Could you check a few things on this drawing? It's one solid part, dimensions in mm from its lowest x, y, z. Round coordinates to 2 decimals unless told otherwise and drop trailing zeros. Write each loop counter-clockwise with the first axis right and the second up, starting at its lowest first coordinate (ties: lowest second). Pieces come first, ordered by that corner, then holes. Notation, with made-up numbers: M -36.5,71 L -4.5,71 A18 cw -4.5,99 Z; hole C 25,30 d11. An arc over 180 degrees is marked long. One line per item, written item: value. Start each with the question number.
(1) I'm going to push a flat-ended pin straight in: pin 1 Ø1 at (x, y) = (15, 1) entering from +Z. Where does the tip first touch, or does it pass through?
(2) I want a section at A-A on x = 26. Please give me the cut outline in (y, z).
(3) If I drill on L1, parallel to Y at x = 20.5, z = 3.6 (3 decimals); L2, parallel to Z at x = 20, y = 2.7, over which ranges is the centre line in solid material (lowest first)?
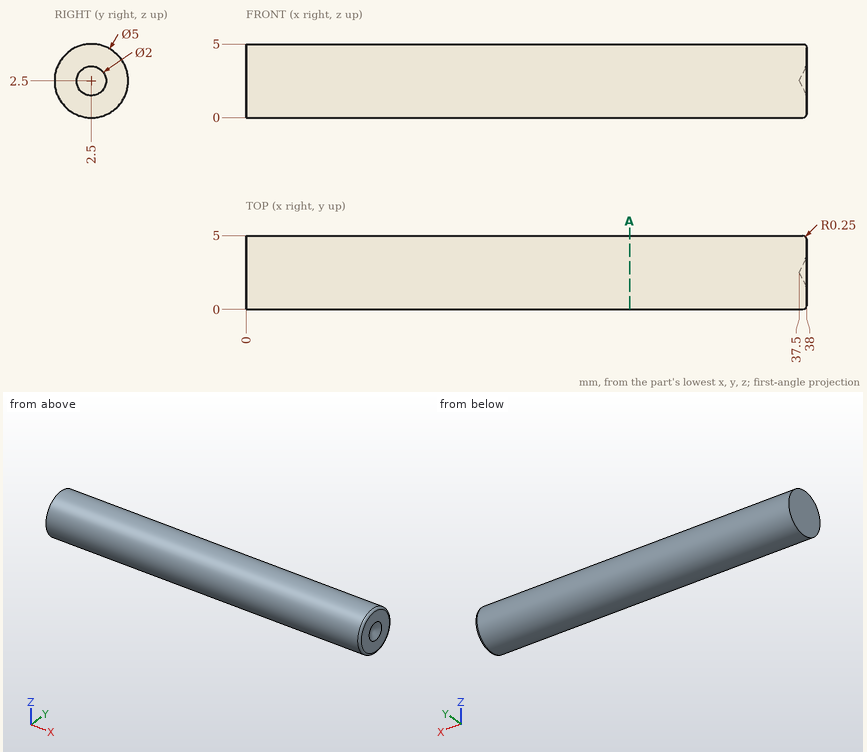
Found:
1. pin 1: stops at z = 4.79
2. outline: C 2.5,2.5 d5
3. L1: y = 0.255 to 4.745
3. L2: z = 0.01 to 4.99
